Can you work these out from the model? Positions are in its coordinate system, mm. Give positions to 0.01 mm unless a question says otherwise; leave off trailing zeros. Loops run counter-clockwise (first coordinate to the right, second up) from the corner with the lowest first, then second, coordinate; pieces in that order, holes last. Notation, with made-up numbers: (9.25, 47) - (46.25, 47) arc R17 ccw to (46.25, 77) - close; hole circle Ø8 at (-13, 0.25). An arc over 180 degrees is marked (long way). Write item = value, one per line.
Autodesk Inventor part; units mm, degrees
ref_plane "YZ Plane" through (0, 0, 0) normal (1, 0, 0) x (0, 1, 0)
ref_plane "XZ Plane" through (0, 0, 0) normal (0, 1, 0) x (-1, 0, 0)
ref_plane "XY Plane" through (0, 0, 0) normal (0, 0, 1) x (1, 0, 0)
sketch "Sketch1" plane through (0, 0, 0) normal (1, 0, 0) x (0, 1, 0)
  line L0 (0, 0) -> (0, -1524)
  line L1 (0, -1524) -> (406.4, -1524)
  line L2 (0, 0) -> (127, 0)
  line L3 (127, 0) -> (406.4, -1524)
  dimension "d0" = 1524
  dimension "d1" = 406.4
  dimension "d2" = 127
extrude "Extrusion1" add sketch "Sketch1" along normal blind 203.2
sketch "Sketch2" plane through (203.2, 0, 0) normal (1, 0, 0) x (0, 0, -1)
  line L0 (0, 0) -> (1524, 0)
  line L1 (1524, 0) -> (1524, 406.4)
  line L2 (1524, 406.4) -> (0, 127)
  line L3 (0, 127) -> (0, 0)
revolve "Revolution1" add sketch "Sketch2" angle 5 about axis through (203.2, 127, 0) along (0, -1, 0)
sketch "Sketch3" plane through (0, 0, 0) normal (-1, 0, 0) x (0, 0, 1)
  line L0 (0, 0) -> (-1524, 0)
  line L1 (0, 127) -> (0, 0)
  line L2 (-1524, 406.4) -> (0, 127)
  line L3 (-1524, 0) -> (-1524, 406.4)
revolve "Revolution2" add sketch "Sketch3" angle 5 about axis through (0, 127, 0) along (0, 1, 0)
properties part number "ramp" material "Wood (Cherry)"
Q1. I need wall thicknesses on L1, parallel to X at y = 49.5, z = -1194; L2, parallel to Y at x = 257, z = -877; L3, parallel to Y at x = 200, z = -386. Which ranges of each line are inside material? Lowest first, please.
Output:
L1 = -104.46 to 307.66
L2 = 0 to 288.09
L3 = 0 to 197.77
Q2. Imagine slicing it at B-B, the plane x = 120. Write out the boundary of the cut face in (y, z), then the cut area to 3 significant figures.
Output:
outline = (0, -1524) - (406.4, -1524) - (127, 0) - (0, 0) - close
area = 406,000 mm2
Q3. For pin 1 (8 mm diameter, centred on x = 287.5, z = -1039.5, fed in from -Y); pin 2 (12 mm diameter, centred on y = 151, z = -948, fed in from -X); pin 3 (1.5 mm diameter, centred on y = 92, z = -1079.5, fed in from +X); pin 4 (6 mm diameter, centred on x = 31, z = -1253.5, fed in from +Y), each with a flat end and sliding along its axis, tell me the tip position at first contact or that it passes through.
Output:
pin_1 = 0
pin_2 = -83.46
pin_3 = 297.71
pin_4 = 357.36
Q4. Imagine slicing it at D-D, the plane y = 375. Write out the boundary of the cut face in (x, z), then the cut area to 3 significant figures.
Output:
outline = (-132.83, -1518.2) arc R1524 ccw to (0, -1524) - (203.2, -1524) arc R1524 ccw to (336.03, -1518.2) - (321.1, -1347.58) arc R1352.73 cw to (203.2, -1352.73) - (0, -1352.73) arc R1352.73 cw to (-117.9, -1347.58) - close
area = 77,800 mm2
Q5. Imagine slicing it at A-A, the plane y = 99. Write out the boundary of the cut face in (x, z), then the cut area to 3 significant figures.
Output:
outline = (-132.83, -1518.2) arc R1524 ccw to (0, -1524) - (203.2, -1524) arc R1524 ccw to (336.03, -1518.2) - (203.2, 0) - (0, 0) - close
area = 512,000 mm2
Q6. Imagine slicing it at C-C, the plane y = 237. Write out the boundary of the cut face in (x, z).
Output:
outline = (-132.83, -1518.2) arc R1524 ccw to (0, -1524) - (203.2, -1524) arc R1524 ccw to (336.03, -1518.2) - (255.49, -597.72) arc R600 cw to (203.2, -600) - (0, -600) arc R600 cw to (-52.29, -597.72) - close
